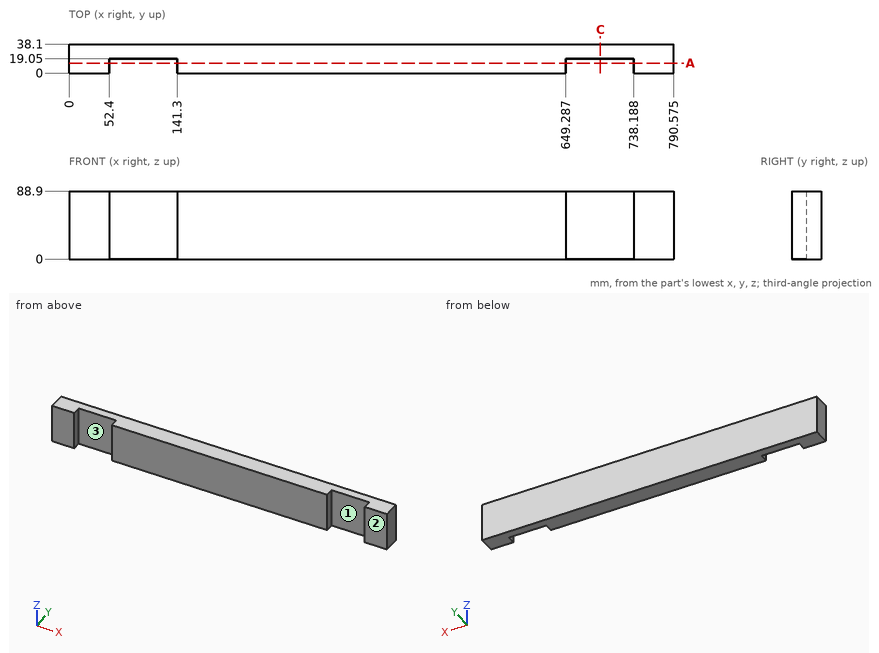
Input: dimensioned drawing with shaded views. Units: mm. Origin: part minimum x, y, z. Give positions to 0.01 mm unless a question says otherwise; leave off trailing zeros. Write each loop counter-clockwise with the first axis right and the second up, starting at its lowest first coordinate (ties: lowest second). Pieces come first, ordered by that corner, then holes. Notation, with made-up numbers: (-2.75, 56) -> (26.25, 56) arc R29 cw to (26.25, 86) -> close; hole circle Ø1 at (73, 17.25). An arc over 180 degrees is marked (long way). Answer as a JSON object with one key per item and string values.
1. Contact query for a flat-ended pin moving along its axis: pin 1 (9.5 mm diameter, centred on y = 7.5, z = 62.5, fed in from -X). Output: stop coordinate, or through.
Ans:
{"pin 1": "stops at x = 0"}
2. Ray query, probe 1 along X at (y, z) = (15.5, 62) (1 decimal); probe 2 along Y at (x, z) = (683, 20). Return the intervals inside material, ascending. Write a range as from..to.
Ans:
{"probe 1": "x = 0..52.4, 141.3..649.3, 738.2..790.6", "probe 2": "y = 19.05..38.1"}
3. Cut plane C-C on x = 694.5. Output: boundary loops of the cut face in (y, z).
Ans:
{"outline": "(19.05, 0) -> (38.1, 0) -> (38.1, 88.9) -> (19.05, 88.9) -> close"}
4. Cut plane A-A on y = 13. Output: boundary loops of the cut face in (x, z) (1 decimal).
Ans:
{"outline": "(0, 0) -> (52.4, 0) -> (52.4, 88.9) -> (0, 88.9) -> close; (141.3, 0) -> (649.3, 0) -> (649.3, 88.9) -> (141.3, 88.9) -> close; (738.2, 0) -> (790.6, 0) -> (790.6, 88.9) -> (738.2, 88.9) -> close"}
5. Mould query, pull axis X, two halves, no side actions, for the marked faces 1, 2 and 3. Classes: pulls with the +X half, pulls with the -X half, needs draft (parallel to the pull), parting line crosses it, or undercut.
Ans:
{"face 1": "undercut", "face 2": "needs draft", "face 3": "undercut"}
